from build123d import *

# Parameters (mm, degrees)
BOSS_EXTRUDE1_START       = -0.25
BOSS_EXTRUDE1_OUTLINE_W   = 22
BOSS_EXTRUDE1_OUTLINE_H   = 0.5
BOSS_EXTRUDE1_OUTLINE_W_2 = 23.5
BOSS_EXTRUDE1_OUTLINE_W_3 = 24.5
BOSS_EXTRUDE1_DEPTH       = 0.5


# Read off the part's stored shape, not the designer's step: Boss-Extrude1
with BuildPart() as part:
    # Sketch1 → Revolve1 (revolve)
    with BuildSketch(Plane.XY, mode=Mode.PRIVATE) as revolve1_sk:
        with BuildLine():
            Line((-6, 0), (-6, -2.95))
            Line((-6, -2.95), (-7, -2.95))
            Line((-7, -2.95), (-7, -2.5))
            Line((-7, -2.5), (-12.1, -2.5))
            ThreePointArc((-12.1, -2.5), (-13.867766953, -1.767766953), (-14.6, 0))
            Line((-14.6, 0), (-6, 0))
        make_face()
    revolve(revolve1_sk.sketch.rotate(Axis((-6, 0, 0), (-1, 0, 0)), 180), axis=Axis((-6, 0, 0), (-1, 0, 0)))

    # Boss-Extrude1 outline → Boss-Extrude1 (add)
    with BuildSketch(Plane.XY.offset(BOSS_EXTRUDE1_START)):
        with Locations((5, -1.855262181)):
            Rectangle(BOSS_EXTRUDE1_OUTLINE_W, BOSS_EXTRUDE1_OUTLINE_H)
        with Locations((5.75, -0.585262181)):
            Rectangle(BOSS_EXTRUDE1_OUTLINE_W_2, BOSS_EXTRUDE1_OUTLINE_H)
        with Locations((6.25, 0.684737819)):
            Rectangle(BOSS_EXTRUDE1_OUTLINE_W_3, BOSS_EXTRUDE1_OUTLINE_H)
        Polygon((16, 2.204737819), (0.47641813, 2.204737819), (0.47641813, 2.547088342), (-1.623745911, 2.547088342), (-1.623745911, 2.204737819), (-6, 2.204737819), (-6, 1.704737819), (-1.623745911, 1.704737819), (-1.623745911, 1.311776605), (0.47641813, 1.311776605), (0.47641813, 1.704737819), (16, 1.704737819), align=None)
    extrude(amount=BOSS_EXTRUDE1_DEPTH)


solid = part.part
Verification items for the finished model (mm, model axes). A direction names the side the tool comes from. Give positions to 0.01 mm unless a question says otherwise; leave off trailing zeros. Order: outer loops, then holes, each group sorted by start corner. A loop starts at its lowest first (then second) coordinate and runs counter-clockwise, first axis right, second up. Notation, with made-up numbers: M 8.5,21.5 L 12.5,21.5 A19 cw 12.5,45.5 Z; hole C 51,27 d10. An arc over 180 degrees is marked long. Use one line per item in the form item = value. Start each with the question number.
Q1. Section check C-C (z = -1.6). Enter the section's corners in (x, y), then the cut area to 3 significant figures.
Q2. Section check B-B (y = 0). Enter the section's corners in (x, z).
Q3. Scan lines: line 1 along Y through (x, z) = (4.5, 0); line 2 along Z through (x, y) = (6, 0.55); line 3 along Z through (x, y) = (-13, -0.25). Record each from-to range of solid material in increasing order. Write a range as [from, to].
Q4. Section check A-A (x = -1). Enter the section's corners in (y, z).
Q5. Access from +Z, -Z, +X, -X, +Y, -Y to the whole of each face (thin tool, end or side, straight path). Record for faces 1 (the flat face through (5, 2, 0.25)), 2 (the cylindrical face through (-9.6, -2.5, -0.1)), 3 (the flat face through (5, 2, -0.25)).
Q6. Go/stop test with flat-tipped pins: pin 1 Ø0.6 at (x, y) = (8, 0.5) entering from +Z; pin 2 Ø0.6 at (x, z) = (-4.5, 0) entering from +Y; pin 3 Ø0.6 at (x, z) = (-3.5, 0) entering from -Y. Record where each tip stops, or that it passes through.
Evaluation:
q1.outline = M -12.1,-1.92 L -7,-1.92 L -7,-2.48 L -6,-2.48 L -6,2.48 L -7,2.48 L -7,1.92 L -12.1,1.92 A1.92 ccw Z
q1.area = 30.3 mm2
q2.outline = M -12.1,-2.5 L -7,-2.5 L -7,-2.95 L -6,-2.95 L -6,2.95 L -7,2.95 L -7,2.5 L -12.1,2.5 A2.5 ccw Z
q3.line_1 = [-2.11, -1.61], [-0.84, -0.34], [0.43, 0.93], [1.7, 2.2]
q3.line_2 = [-0.25, 0.25]
q3.line_3 = [-2.32, 2.32]
q4.outline = M -2.11,-0.25 L -1.61,-0.25 L -1.61,0.25 L -2.11,0.25 Z; M -0.84,-0.25 L -0.34,-0.25 L -0.34,0.25 L -0.84,0.25 Z; M 0.43,-0.25 L 0.93,-0.25 L 0.93,0.25 L 0.43,0.25 Z; M 1.31,-0.25 L 2.55,-0.25 L 2.55,0.25 L 1.31,0.25 Z
q5.face_1 = +Z, +X, +Y, -Y
q5.face_2 = -X
q5.face_3 = -Z, +X, +Y, -Y
q6.pin_1 = 0.25
q6.pin_2 = 2.2
q6.pin_3 = -2.11
